Geometry check sheet. Reference: drawing and pictorial views, mm from the part's lowest x, y, z. A direction names the side the tool comes from. Round coordinates to 2 decimals unless told otherwise and drop trailing zeros. Write each loop counter-clockwise with the first axis right and the second up, starting at its lowest first coordinate (ties: lowest second). Pieces come first, ordered by that corner, then holes. Notation, with made-up numbers: M 43,45.25 L 48,45.25 A22 cw 48,52.25 Z; hole C 79,69 d4. An arc over 180 degrees is marked long. Answer in a Markdown table with one row per item. Add a question column.
1. Go/stop test with flat-tipped pins: pin 1 Ø3.5 at (x, y) = (12.75, 7.62) entering from -Z; pin 2 Ø3 at (x, y) = (5.5, 19) entering from +Z. Record where each tip stops, or that it passes through.
2. Draft check along X on the marked faces 1, 2 and 3. Enter one of: pulls with the +X half, pulls with the -X half, needs draft (parallel to the pull), parting line crosses it, or undercut.
3. Set-up check for the marked faces 4 and 5: record each of +Z, -Z, +X, -X, +Y, -Y from which the full face is reachable in a straight line by a thin tool's end or side.
4. Sectioned sample at A-A on z = 39. Record the cut outline in (x, y).
5. Sectioned sample at D-D on z = 11.5. Record the cut outline in (x, y) (1 decimal).
6. Sectioned sample at B-B on y = 7.62. Record the cut outline in (x, z) (1 decimal), plus the area to 3 significant figures.
7. Sectioned sample at C-C on x = 41. Record the cut outline in (y, z) (1 decimal).
8. Material ranges on probe 1 along X at (y, z) = (7, 30); probe 2 along X at (y, z) = (4, 52.5); probe 3 along Z at (x, y) = (4, 35.5), recorded low to high.
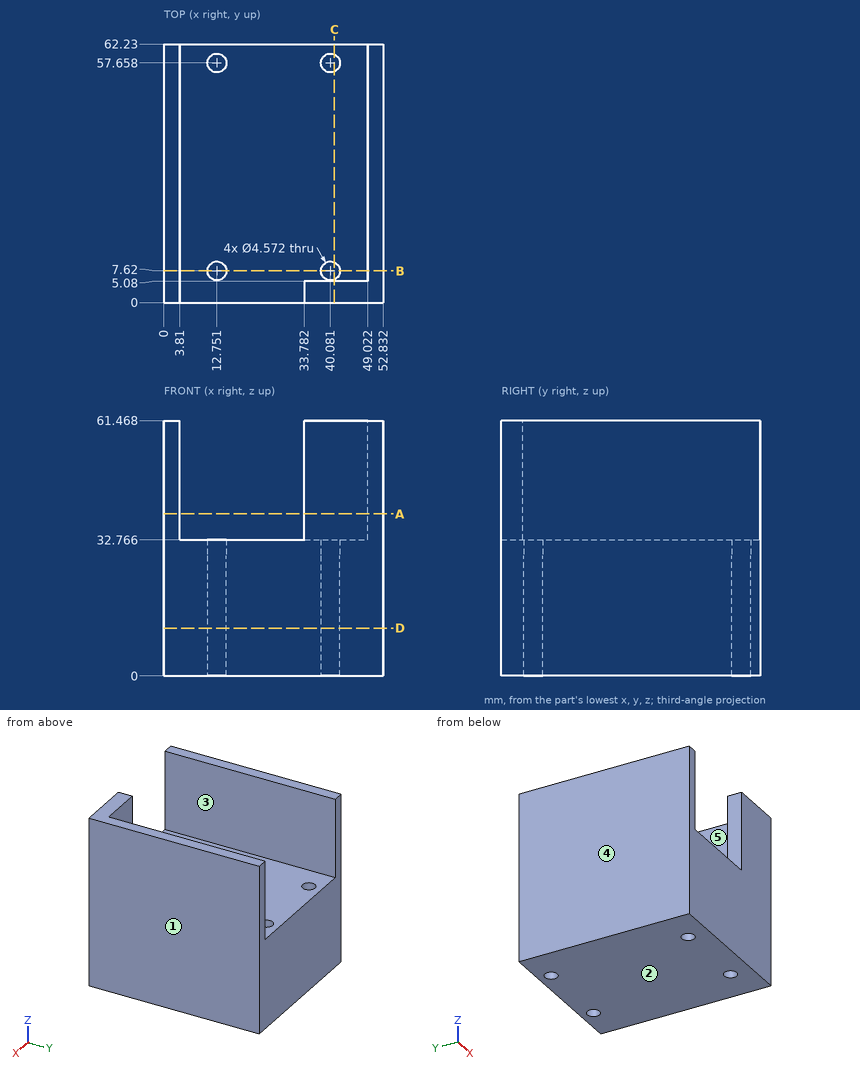
Geometry check:
| question | item | result |
|---|---|---|
| 1 | pin 1 | passes through |
| 1 | pin 2 | stops at z = 32.77 |
| 2 | face 1 | pulls with the +X half |
| 2 | face 2 | needs draft |
| 2 | face 3 | undercut |
| 3 | face 4 | +Z, -Z, -X, +Y, -Y |
| 3 | face 5 | +Z, +Y |
| 4 | outline | M 0,0 L 3.81,0 L 3.81,62.23 L 0,62.23 Z; M 33.78,0 L 52.83,0 L 52.83,62.23 L 49.02,62.23 L 49.02,5.08 L 33.78,5.08 Z |
| 5 | outline | M 0,0 L 52.8,0 L 52.8,62.2 L 0,62.2 Z; hole C 12.8,7.6 d4.6; hole C 12.8,57.7 d4.6; hole C 40.1,7.6 d4.6; hole C 40.1,57.7 d4.6 |
| 6 | outline | M 0,0 L 10.5,0 L 10.5,32.8 L 3.8,32.8 L 3.8,61.5 L 0,61.5 Z; M 15,0 L 37.8,0 L 37.8,32.8 L 15,32.8 Z; M 42.4,0 L 52.8,0 L 52.8,61.5 L 49,61.5 L 49,32.8 L 42.4,32.8 Z |
| 6 | area | 1,650 mm2 |
| 7 | outline | M 0,0 L 5.5,0 L 5.5,32.8 L 5.1,32.8 L 5.1,61.5 L 0,61.5 Z; M 9.7,0 L 55.6,0 L 55.6,32.8 L 9.7,32.8 Z; M 59.8,0 L 62.2,0 L 62.2,32.8 L 59.8,32.8 Z |
| 8 | probe 1 | x = 0 to 10.55, 14.95 to 37.88, 42.28 to 52.83 |
| 8 | probe 2 | x = 0 to 3.81, 33.78 to 52.83 |
| 8 | probe 3 | z = 0 to 32.77 |
